Geometry: final body of the model. Coordinates: model frame, mm. Face numbers are marked on the shaded views. A direction names the side the tool comes from. Give positions to 0.01 mm unless a question says otherwise; leave off trailing zeros. Loops run counter-clockwise (first coordinate to the right, second up) from the corner with the lowest first, then second, coordinate; pieces in that order, holes last.
from build123d import *

# Parameters (mm, degrees)
F0_R            = 317.5
F0_R_2          = 127
F1_DEPTH        = 76.2
F3_DEPTH        = 254
F4_R            = 12.7
F6_DEPTH        = 330.2
F7_R            = 25.4
F8_DEPTH        = 76.201
F8_COPIES_COUNT = 4


# Not quite as in the source:
# - a pattern or mirror of a feature is missing from the dataset's text; its kind, count and spacing are read off the source's solid


with BuildPart() as f1:
    # F0 (on Top) → F1 (new body)
    with BuildSketch(Plane.XY):
        Circle(F0_R)
        Circle(F0_R_2, mode=Mode.SUBTRACT)
    extrude(amount=F1_DEPTH)

    # F2 (on face) → F3 (join)
    with BuildSketch(Plane.XY.offset(76.2)):
        with BuildLine():
            ThreePointArc((-241.9674978174, 139.7), (0, 279.4), (241.9674978174, 139.7))
            Line((241.9674978174, 139.7), (274.9630657016, 158.75))
            ThreePointArc((274.9630657016, 158.75), (0, 317.5), (-274.9630657016, 158.75))
            Line((-274.9630657016, 158.75), (-241.9674978174, 139.7))
        make_face()
    extrude(amount=F3_DEPTH)

    # F4
    f4_edges = [f1.edges().sort_by_distance(p)[0] for p in [
        (-274.963066, 158.75, 203.2),
        (-241.967498, 139.7, 203.2),
        (241.967498, 139.7, 203.2),
        (274.963066, 158.75, 203.2),
    ]]
    fillet(f4_edges, radius=F4_R)

    # F5 (on face) → F6 (join, through all)
    with BuildSketch(Plane.XY.offset(330.2)):
        with BuildLine():
            ThreePointArc((25.3796718655, 316.484), (25.3949174579, 316.9918983288), (25.4, 317.5))
            ThreePointArc((25.4, 317.5), (-0.5081016712, 342.8949174579), (-25.3796718655, 316.484))
            ThreePointArc((-25.3796718655, 316.484), (0, 317.5), (25.3796718655, 316.484))
        make_face()
        with BuildLine():
            ThreePointArc((25.3796718655, 316.484), (0, 317.5), (-25.3796718655, 316.484))
            ThreePointArc((-25.3796718655, 316.484), (0, 292.1), (25.3796718655, 316.484))
        make_face()
    extrude(amount=-F6_DEPTH)

    # F7 (on face) → F8 (cut, through all)
    with BuildSketch(Plane.XY.offset(76.2)):
        with Locations((-203.2, 0)):
            Circle(F7_R)
    f8 = extrude(amount=-F8_DEPTH, mode=Mode.SUBTRACT)

    # F8_copies: F8 ×4 about axis
    f8_copies_axis = Axis((0, 0, 0), (0, 0, 1))
    for i in range(1, F8_COPIES_COUNT):
        add(f8.rotate(f8_copies_axis, i * 360 / F8_COPIES_COUNT), mode=Mode.SUBTRACT)


solid = f1.part
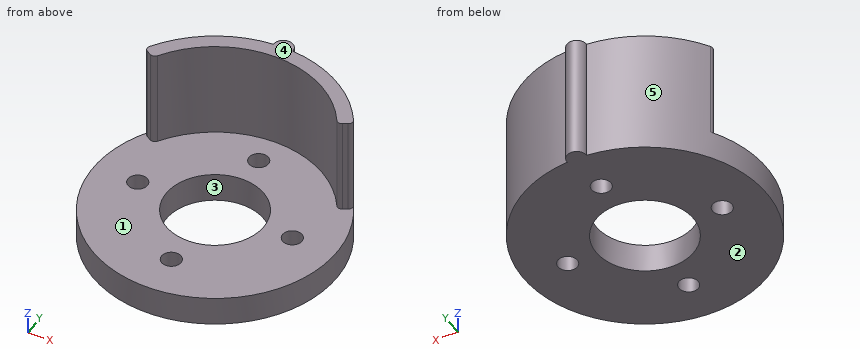
Item 1: Set-up query: the marked faces 1 and 2. Return all of +Z, -Z, +X, -X, +Y, -Y with unobstructed straight access to the full face (end or side cutting, diameter ignored); none if empty.
Values follow:
face 1: +Z, -Y
face 2: -Z, +X, -X, +Y, -Y
Item 2: Draft query along X for the marked faces 3, 4 and 5. Return one class per face: +X half, -X half, draft (parallel to the pull), parting line (faces both ways), or undercut.
Values follow:
face 3: undercut
face 4: draft
face 5: parting line
Item 3: Ray query, probe 1 along Z at (x, y) = (118, 121); probe 2 along X at (y, z) = (-203, 27); probe 3 along X at (y, z) = (129.5, 50.5). Return the intervals inside material, ascending.
Values follow:
probe 1: z = 0 to 76.2
probe 2: x = -244.13 to -25.4, 25.4 to 244.13
probe 3: x = -289.89 to 289.89
Item 4: Section query B-B on x = 0. Return loops of the section in (y, z), plus the area to 3 significant figures.
Values follow:
outline: (-317.5, 0) - (-228.6, 0) - (-228.6, 76.2) - (-317.5, 76.2) - close; (-177.8, 0) - (-127, 0) - (-127, 76.2) - (-177.8, 76.2) - close; (127, 0) - (177.8, 0) - (177.8, 76.2) - (127, 76.2) - close; (228.6, 0) - (342.9, 0) - (342.9, 330.2) - (279.4, 330.2) - (279.4, 76.2) - (228.6, 76.2) - close
area: 39,400 mm2
Item 5: Section query C-C on x = 203.2. Return loops of the section in (y, z), plus the area to 3 significant figures.
Values follow:
outline: (-243.96, 0) - (-25.4, 0) - (-25.4, 76.2) - (-243.96, 76.2) - close; (25.4, 0) - (243.96, 0) - (243.96, 330.2) - (191.77, 330.2) - (191.77, 76.2) - (25.4, 76.2) - close
area: 46,600 mm2
Item 6: Section query A-A on y = 0. Return loops of the section in (x, z), plus the area to 3 significant figures.
Values follow:
outline: (-317.5, 0) - (-228.6, 0) - (-228.6, 76.2) - (-317.5, 76.2) - close; (-177.8, 0) - (-127, 0) - (-127, 76.2) - (-177.8, 76.2) - close; (127, 0) - (177.8, 0) - (177.8, 76.2) - (127, 76.2) - close; (228.6, 0) - (317.5, 0) - (317.5, 76.2) - (228.6, 76.2) - close
area: 21,300 mm2
Item 7: Section query D-D on y = 203.2. Return loops of the section in (x, z), plus the area to 3 significant figures.
Values follow:
outline: (-243.96, 0) - (-25.4, 0) - (-25.4, 76.2) - (-191.77, 76.2) - (-191.77, 330.2) - (-243.96, 330.2) - close; (25.4, 0) - (243.96, 0) - (243.96, 330.2) - (191.77, 330.2) - (191.77, 76.2) - (25.4, 76.2) - close
area: 59,800 mm2
Item 8: Pin query (flat end, axial travel): pin 1 (10 mm diameter, centred on x = -164.5, y = 89, fed in from +Z); pin 2 (1 mm diameter, centred on x = -114, z = 173.5, fed in from +Y); pin 3 (1 mm diameter, centred on x = -129, z = 282, fed in from +Y). Return the tip coordinate at first contact, or that it passes through.
Values follow:
pin 1: stops at z = 76.2
pin 2: stops at y = 296.52
pin 3: stops at y = 290.33
